Can you work these out from the model? Positions are in its coordinate system, mm. Face numbers are marked on the shaded views. A direction names the side the tool comes from. Round coordinates to 2 decimals unless told otherwise and drop trailing zeros. Loops run counter-clockwise (first coordinate to the right, second up) from the corner with the lowest first, then second, coordinate; pieces in that order, holes last.
(1) I want a section at D-D on y = -19.5. Write out the boundary of the cut face in (x, z), plus the area to 3 significant figures.
(2) I want a section at A-A on z = -11.5. Write out the boundary of the cut face in (x, y).
(3) I want a section at B-B on z = -3. Write out the boundary of the cut face in (x, y).
(4) Will these pins go through, and if not, where does the flat tip stop? pin 1 Ø5 at (x, y) = (10.5, 13) entering from -Z; pin 2 Ø3.5 at (x, y) = (9.775, 13.7) entering from +Z; pin 3 Ø4.5 at (x, y) = (-19.6, 0) entering from +Z; pin 4 Ø1.5 at (x, y) = (-25, 4.5) entering from -Z.
(5) Thinking about a two-plate mould opening in X: for the marked faces 1, 2 and 3, which applies, released by +X, released by -X, zero draft, split by the parting line, or undercut?
(6) I want a section at C-C on x = -46.5. Write out the boundary of the cut face in (y, z).
(7) If I drill on line 1 along X through (y, z) = (13.7, 3) (3 decimals); line 2 along Y through (x, z) = (-19.6, -8.25); line 3 along Y through (x, z) = (-19.6, -3.75), over which ranges is the centre line in solid material (lowest first)?
(8) Which directions (+Z, -Z, +X, -X, +Y, -Y) give clear straight access to the entire face, cutting with the end or side of a thin tool? Please do the marked faces 4 and 5.
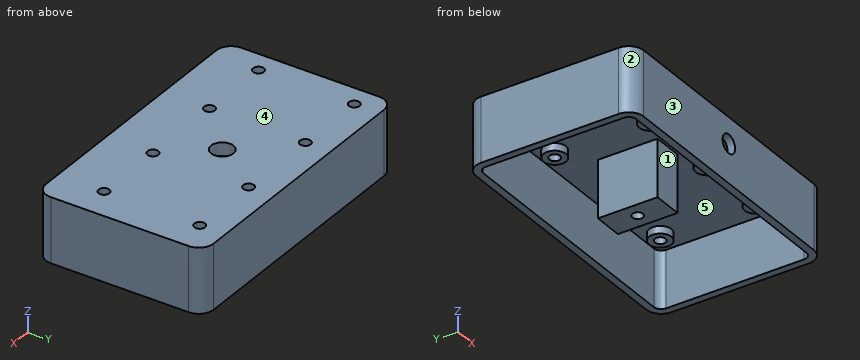
Autodesk Inventor part; units mm, degrees
ref_plane "Work Plane3" through (-11.0937, -12.5187, -13.35) normal (0, 0, 1) x (1, 0, 0)
ref_plane "YZ Plane" through (0, 0, 0) normal (1, 0, 0) x (0, 1, 0)
ref_plane "XZ Plane" through (0, 0, 0) normal (0, 1, 0) x (-1, 0, 0)
ref_plane "Work Plane1" through (0, 0, 0) normal (0, 0, 1) x (1, 0, 0)
ref_plane "Work Plane2" through (0, 0, 2) normal (0, 0, 1) x (1, 0, 0)
sketch "Sketch1" plane through (0, 0, 2) normal (0, 0, 1) x (1, 0, 0)
  circle A0 centre (9.775, 13.7) radius 1.45 construction
  circle A1 centre (-9.775, 13.7) radius 1.45 construction
  circle A2 centre (9.775, -12) radius 1.45 construction
  circle A3 centre (-9.775, -12) radius 1.45 construction
  line L0 (-13.075, -17) -> (13.075, -17) construction
  line L1 (13.075, -17) -> (13.075, 17) construction
  line L2 (13.075, 17) -> (-13.075, 17) construction
  line L3 (-13.075, 17) -> (-13.075, -17) construction
  circle A4 centre (-32.375, 13.7) radius 1.45 construction
  circle A5 centre (-51.925, 13.7) radius 1.45 construction
  circle A6 centre (-32.375, -12) radius 1.45 construction
  circle A7 centre (-51.925, -12) radius 1.45 construction
  line L4 (-55.225, -17) -> (-29.075, -17) construction
  line L5 (-29.075, -17) -> (-29.075, 17) construction
  line L6 (-29.075, 17) -> (-55.225, 17) construction
  line L7 (-55.225, 17) -> (-55.225, -17) construction
  line L8 (18.4, -24.45) -> (-57.6, -24.45) construction
  line L9 (-57.6, -24.45) -> (-57.6, 20.55) construction
  line L10 (-57.6, 20.55) -> (18.4, 20.55) construction
  line L11 (18.4, 20.55) -> (18.4, -24.45) construction
  line L12 (18.4, -24.45) -> (-57.6, 20.55) construction
  line L13 (-57.6, -24.45) -> (18.4, 20.55) construction
  line L14 (18.4, 20.55) -> (-57.6, 20.55)
  line L15 (-57.6, 20.55) -> (-57.6, -24.45)
  line L16 (-57.6, -24.45) -> (18.4, -24.45)
  line L17 (18.4, -24.45) -> (18.4, 20.55)
  circle A8 centre (1.475, 0.05) radius 3.625
  circle A9 centre (-40.675, 0.05) radius 3.625
  point P0 (0, 0)
  point P1 (-19.6, -1.95)
  dimension "d0" = 76
  dimension "d1" = 45
  dimension "d2" = 42.15
  dimension "d3" = 21.075
  dimension "d24" = 2
extrude "Extrusion1" add sketch "Sketch1" along normal blind 2 contours L17 L16 L15 L14 | A8 | A9
sketch "Sketch2" plane through (0, 0, 2) normal (0, 0, -1) x (-1, 0, 0)
  line L0 (48.625, -15.2642) -> (36.125, -15.2642)
  line L1 (36.125, -15.2642) -> (36.125, -13.7335)
  line L2 (36.125, -13.7335) -> (48.625, -13.7335)
  line L3 (48.625, -13.7335) -> (48.625, -15.2642)
  line L4 (55.225, -17) -> (29.075, -17)
  line L5 (55.225, 17) -> (55.225, -17)
  line L6 (29.075, 17) -> (55.225, 17)
  line L7 (29.075, -17) -> (29.075, 17)
  circle A0 centre (51.925, -12) radius 1.45
  circle A1 centre (32.375, -12) radius 1.45
  circle A2 centre (51.925, 13.7) radius 1.45
  circle A3 centre (32.375, 13.7) radius 1.45
  line L8 (48.025, 8.1) -> (33.325, 8.1)
  arc A4 (48.725, 7.4) -> (48.025, 8.1) centre (48.025, 7.4) ccw
  line L9 (48.725, 3.55) -> (48.725, 7.4)
  line L10 (47.725, 3.55) -> (48.725, 3.55)
  line L11 (47.725, -3.45) -> (47.725, 3.55)
  line L12 (47.725, -3.45) -> (48.725, -3.45)
  line L13 (48.725, -7.3) -> (48.725, -3.45)
  arc A5 (48.025, -8) -> (48.725, -7.3) centre (48.025, -7.3) ccw
  line L14 (33.325, -8) -> (48.025, -8)
  arc A6 (32.625, -7.3) -> (33.325, -8) centre (33.325, -7.3) ccw
  line L15 (32.625, 7.4) -> (32.625, -7.3)
  arc A7 (33.325, 8.1) -> (32.625, 7.4) centre (33.325, 7.4) ccw
  circle A8 centre (51.925, 13.7) radius 3
  circle A9 centre (51.925, -12) radius 3
  circle A10 centre (32.375, -12) radius 3
  circle A11 centre (32.375, 13.7) radius 3
  line L16 (6.475, -15.2642) -> (-6.025, -15.2642)
  line L17 (-6.025, -15.2642) -> (-6.025, -13.7335)
  line L18 (-6.025, -13.7335) -> (6.475, -13.7335)
  line L19 (6.475, -13.7335) -> (6.475, -15.2642)
  line L20 (13.075, -17) -> (-13.075, -17)
  line L21 (13.075, 17) -> (13.075, -17)
  line L22 (-13.075, 17) -> (13.075, 17)
  line L23 (-13.075, -17) -> (-13.075, 17)
  circle A12 centre (9.775, -12) radius 1.45
  circle A13 centre (-9.775, -12) radius 1.45
  circle A14 centre (9.775, 13.7) radius 1.45
  circle A15 centre (-9.775, 13.7) radius 1.45
  line L24 (5.875, 8.1) -> (-8.825, 8.1)
  arc A16 (6.575, 7.4) -> (5.875, 8.1) centre (5.875, 7.4) ccw
  line L25 (6.575, 3.55) -> (6.575, 7.4)
  line L26 (5.575, 3.55) -> (6.575, 3.55)
  line L27 (5.575, -3.45) -> (5.575, 3.55)
  line L28 (5.575, -3.45) -> (6.575, -3.45)
  line L29 (6.575, -7.3) -> (6.575, -3.45)
  arc A17 (5.875, -8) -> (6.575, -7.3) centre (5.875, -7.3) ccw
  line L30 (-8.825, -8) -> (5.875, -8)
  arc A18 (-9.525, -7.3) -> (-8.825, -8) centre (-8.825, -7.3) ccw
  line L31 (-9.525, 7.4) -> (-9.525, -7.3)
  arc A19 (-8.825, 8.1) -> (-9.525, 7.4) centre (-8.825, 7.4) ccw
  circle A20 centre (9.775, 13.7) radius 3
  circle A21 centre (9.775, -12) radius 3
  circle A22 centre (-9.775, -12) radius 3
  circle A23 centre (-9.775, 13.7) radius 3
  point P0 (0, 0)
  dimension "d6" = 6
  dimension "d7" = 6
  dimension "d8" = 6
  dimension "d9" = 6
  dimension "d10" = 6
  dimension "d11" = 6
  dimension "d12" = 6
  dimension "d13" = 6
extrude "Extrusion2" add sketch "Sketch2" along normal blind 2 contours A8 | A9 | A10 | A11 | A20 | A21 | A22 | A23
fillet "Fillet1" radius 4 4 edges at (18.4, 20.55, 3) (18.4, -24.45, 3) (-57.6, -24.45, 3) (-57.6, 20.55, 3)
sketch "Sketch3" plane through (0, 0, 2) normal (0, 0, -1) x (-1, 0, 0)
  circle A0 centre (-9.775, -12) radius 3
  circle A1 centre (9.775, 13.7) radius 3
  circle A2 centre (32.375, -12) radius 3
  circle A3 centre (51.925, 13.7) radius 3
  circle A4 centre (51.925, -12) radius 3
  circle A5 centre (32.375, 13.7) radius 3
  circle A6 centre (9.775, -12) radius 3
  circle A7 centre (-9.775, 13.7) radius 3
  arc A8 (57.6, 16.55) -> (53.6, 20.55) centre (53.6, 16.55) ccw
  line L0 (53.6, 20.55) -> (-14.4, 20.55)
  arc A9 (-14.4, 20.55) -> (-18.4, 16.55) centre (-14.4, 16.55) ccw
  line L1 (-18.4, 16.55) -> (-18.4, -20.45)
  arc A10 (-18.4, -20.45) -> (-14.4, -24.45) centre (-14.4, -20.45) ccw
  line L2 (-14.4, -24.45) -> (53.6, -24.45)
  arc A11 (53.6, -24.45) -> (57.6, -20.45) centre (53.6, -20.45) ccw
  line L3 (57.6, -20.45) -> (57.6, 16.55)
  point P0 (0, 0)
hole "Hole1" at (-51.925, 13.7, 2) at (-51.925, -12, 2) at (-32.375, -12, 2) at (-32.375, 13.7, 2) at (-9.775, 13.7, 2) at (9.775, 13.7, 2) at (-9.775, -12, 2) at (9.775, -12, 2) direction (0, 0, 1) diameter 2.9 end through all
ref_plane "Work Plane3" through (-11.0937, -12.5187, -13.35) normal (0, 0, 1) x (1, 0, 0)
sketch "Sketch4" plane through (0, 0, 2) normal (0, 0, -1) x (-1, 0, 0)
  circle A0 centre (-9.775, -12) radius 3
  circle A1 centre (9.775, 13.7) radius 3
  circle A2 centre (32.375, -12) radius 3
  circle A3 centre (51.925, 13.7) radius 3
  circle A4 centre (51.925, -12) radius 3
  circle A5 centre (32.375, 13.7) radius 3
  circle A6 centre (9.775, -12) radius 3
  circle A7 centre (-9.775, 13.7) radius 3
  arc A8 (57.6, 16.55) -> (53.6, 20.55) centre (53.6, 16.55) ccw
  line L0 (53.6, 20.55) -> (-14.4, 20.55)
  arc A9 (-14.4, 20.55) -> (-18.4, 16.55) centre (-14.4, 16.55) ccw
  line L1 (-18.4, 16.55) -> (-18.4, -20.45)
  arc A10 (-18.4, -20.45) -> (-14.4, -24.45) centre (-14.4, -20.45) ccw
  line L2 (-14.4, -24.45) -> (53.6, -24.45)
  arc A11 (53.6, -24.45) -> (57.6, -20.45) centre (53.6, -20.45) ccw
  line L3 (57.6, -20.45) -> (57.6, 16.55)
  arc A12 (55.6, 16.55) -> (53.6, 18.55) centre (53.6, 16.55) ccw
  line L4 (53.6, 18.55) -> (-14.4, 18.55)
  arc A13 (-14.4, 18.55) -> (-16.4, 16.55) centre (-14.4, 16.55) ccw
  line L5 (-16.4, 16.55) -> (-16.4, -20.45)
  arc A14 (-16.4, -20.45) -> (-14.4, -22.45) centre (-14.4, -20.45) ccw
  line L6 (-14.4, -22.45) -> (53.6, -22.45)
  arc A15 (53.6, -22.45) -> (55.6, -20.45) centre (53.6, -20.45) ccw
  line L7 (55.6, -20.45) -> (55.6, 16.55)
  point P0 (0, 0)
  dimension "d25" = 2
extrude "Extrusion3" add sketch "Sketch4" along normal up to surface (15.35 mm away) contours L3 A11 L2 A10 L1 A9 L0 A8
sketch "Sketch5" plane through (-53.6, -24.45, 4) normal (0, -1, 0) x (1, 0, 0)
  line L0 (0, -17.35) -> (0, 0)
  line L1 (68, 0) -> (68, -17.35)
  line L2 (0, 0) -> (68, 0)
  circle A0 centre (34, -7) radius 2.5
  line L3 (68, -17.35) -> (0, -17.35)
  point P0 (53.6, -4)
  dimension "d28" = 5
extrude "Extrusion4" cut sketch "Sketch5" against normal blind 12 contours A0
sketch "Sketch6" plane through (0, 0, -13.35) normal (0, 0, -1) x (-1, 0, 0)
  line L0 (55.6, 16.55) -> (55.6, -20.45)
  arc A0 (53.6, -22.45) -> (55.6, -20.45) centre (53.6, -20.45) ccw
  line L1 (53.6, -22.45) -> (-14.4, -22.45)
  arc A1 (-16.4, -20.45) -> (-14.4, -22.45) centre (-14.4, -20.45) ccw
  line L2 (-16.4, -20.45) -> (-16.4, 16.55)
  arc A2 (-14.4, 18.55) -> (-16.4, 16.55) centre (-14.4, 16.55) ccw
  line L3 (-14.4, 18.55) -> (53.6, 18.55)
  arc A3 (55.6, 16.55) -> (53.6, 18.55) centre (53.6, 16.55) ccw
  arc A4 (57.6, 16.55) -> (53.6, 20.55) centre (53.6, 16.55) ccw
  line L4 (53.6, 20.55) -> (-14.4, 20.55)
  arc A5 (-14.4, 20.55) -> (-18.4, 16.55) centre (-14.4, 16.55) ccw
  line L5 (-18.4, 16.55) -> (-18.4, -20.45)
  arc A6 (-18.4, -20.45) -> (-14.4, -24.45) centre (-14.4, -20.45) ccw
  line L6 (-14.4, -24.45) -> (53.6, -24.45)
  arc A7 (53.6, -24.45) -> (57.6, -20.45) centre (53.6, -20.45) ccw
  line L7 (57.6, -20.45) -> (57.6, 16.55)
  line L8 (15.6, 8) -> (23.6, 8)
  line L9 (23.6, 8) -> (23.6, -8)
  line L10 (23.6, -8) -> (15.6, -8)
  line L11 (15.6, -8) -> (15.6, 8)
  line L12 (15.6, 8) -> (23.6, -8) construction
  line L13 (23.6, 8) -> (15.6, -8) construction
  point P0 (0, 0)
  point P1 (19.6, 0)
  dimension "d31" = 8
  dimension "d32" = 16
extrude "Extrusion5" add sketch "Sketch6" against normal up to next contours L8 L9 L10 L11
sketch "Sketch7" plane through (0, 0, 4) normal (0, 0, 1) x (1, 0, 0)
  line L0 (-15.6, 8) -> (-23.6, 8)
  line L1 (-15.6, -8) -> (-15.6, 8)
  line L2 (-23.6, -8) -> (-15.6, -8)
  line L3 (-23.6, 8) -> (-23.6, -8)
  circle A0 centre (-19.6, 0) radius 1.5839
  point P0 (0, 0)
hole "Hole2" at (-19.6, 0, 4) direction (0, 0, -1) diameter 2.9 end through all counterbore diameter 6 counterbore depth 3.5
properties part number "40_Joystick_PS2_Base"
Filled sheet:
1. outline: (-57.6, -13.35) - (-55.6, -13.35) - (-55.6, 2) - (16.4, 2) - (16.4, -13.35) - (18.4, -13.35) - (18.4, 4) - (-57.6, 4) - close
1. area: 213 mm2
2. outline: (-57.6, -20.45) arc R4 ccw to (-53.6, -24.45) - (14.4, -24.45) arc R4 ccw to (18.4, -20.45) - (18.4, 16.55) arc R4 ccw to (14.4, 20.55) - (-53.6, 20.55) arc R4 ccw to (-57.6, 16.55) - close; (-23.6, -8) - (-15.6, -8) - (-15.6, 8) - (-23.6, 8) - close; hole (-55.6, -20.45) arc R2 ccw to (-53.6, -22.45) - (14.4, -22.45) arc R2 ccw to (16.4, -20.45) - (16.4, 16.55) arc R2 ccw to (14.4, 18.55) - (-53.6, 18.55) arc R2 ccw to (-55.6, 16.55) - close; hole circle Ø2.9 at (-19.6, 0)
3. outline: (-57.6, -20.45) arc R4 ccw to (-53.6, -24.45) - (-22.1, -24.45) - (-22.1, -22.45) - (-53.6, -22.45) arc R2 cw to (-55.6, -20.45) - (-55.6, 16.55) arc R2 cw to (-53.6, 18.55) - (14.4, 18.55) arc R2 cw to (16.4, 16.55) - (16.4, -20.45) arc R2 cw to (14.4, -22.45) - (-17.1, -22.45) - (-17.1, -24.45) - (14.4, -24.45) arc R4 ccw to (18.4, -20.45) - (18.4, 16.55) arc R4 ccw to (14.4, 20.55) - (-53.6, 20.55) arc R4 ccw to (-57.6, 16.55) - close; (-23.6, -8) - (-15.6, -8) - (-15.6, 8) - (-23.6, 8) - close; hole circle Ø2.9 at (-19.6, 0)
4. pin 1: stops at z = 0
4. pin 2: stops at z = 4
4. pin 3: stops at z = 0.5
4. pin 4: stops at z = 2
5. face 1: undercut
5. face 2: released by -X
5. face 3: zero draft
6. outline: (-24.45, -13.35) - (-22.45, -13.35) - (-22.45, 2) - (18.55, 2) - (18.55, -13.35) - (20.55, -13.35) - (20.55, 4) - (-24.45, 4) - close
7. line 1: x = -57.6 to -53.375, -50.475 to -33.825, -30.925 to -11.225, -8.325 to 8.325, 11.225 to 18.4
7. line 2: y = -24.45 to -22.45, -8 to -1.45, 1.45 to 8, 18.55 to 20.55
7. line 3: y = -8 to -1.45, 1.45 to 8, 18.55 to 20.55
8. face 4: +Z, +X, -X, +Y, -Y
8. face 5: -Z
